Can you work these out from the model? Positions are in its coordinate system, mm. Face numbers are marked on the shaded views. Give positions to 0.01 mm unless a question says otherwise; leave off trailing zeros. Order: outer loops, then holes, each group sorted by start corner. A loop starts at its lowest first (then second) coordinate and runs counter-clockwise, first axis right, second up. Notation, with made-up numbers: M -31.5,-22.5 L -12.5,-22.5 A28 cw -12.5,-2.5 Z; hole C 47.5,-40 d6. An arc over 180 degrees is marked long. Write each question's results on one line, items separated by ' | '.
from build123d import *

# Parameters (mm, degrees)
SKETCH1_R               = 12
BOSS_EXTRUDE1_DEPTH     = 114.25
SKETCH2_R               = 11.565
CUT_EXTRUDE1_DEPTH      = 40
SKETCH3_R               = 3.3
CUT_EXTRUDE2_DEPTH      = 1
CUT_EXTRUDE2_DEPTH_BACK = 115.25


with BuildPart() as part:
    # Sketch1 → Boss-Extrude1 (new body)
    with BuildSketch(Plane(origin=(0, 0, 0), x_dir=(1, 0, 0), z_dir=(0, 1, 0))):
        Circle(SKETCH1_R)
    extrude(amount=BOSS_EXTRUDE1_DEPTH)

    # Sketch2 → Cut-Extrude1 (cut)
    with BuildSketch(Plane(origin=(0, 114.25, 0), x_dir=(1, 0, 0), z_dir=(0, 1, 0))):
        Circle(SKETCH2_R)
    extrude(amount=-CUT_EXTRUDE1_DEPTH, mode=Mode.SUBTRACT)

    # Sketch3 → Cut-Extrude2 (cut, two sides)
    with BuildSketch(Plane.XZ) as cut_extrude2_sk:
        Circle(SKETCH3_R)
    extrude(amount=CUT_EXTRUDE2_DEPTH, mode=Mode.SUBTRACT)
    extrude(cut_extrude2_sk.sketch, amount=-CUT_EXTRUDE2_DEPTH_BACK, mode=Mode.SUBTRACT)


solid = part.part
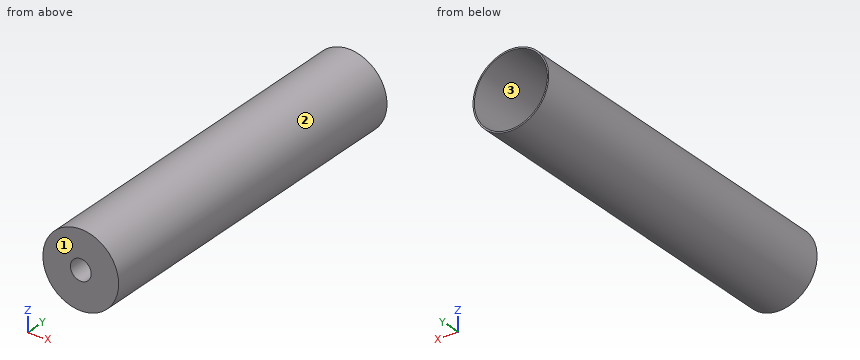
(1) I need wall thicknesses on L1, parallel to X at y = 100, z = 0 (3 decimals); L2, parallel to Y at x = -3.75, z = -6.75. Which ranges of each line are inside material? Lowest first, please. Write a range as from..to.
Data:
L1: x = -12..-11.565, 11.565..12 | L2: y = 0..74.25
(2) Imagine slicing it at C-C, the plane y = 79.5. Write out the boundary of the cut face in (x, z) (3 decimals), plus the area to 3 significant figures.
Data:
outline: C 0,0 d24; hole C 0,0 d23.13 | area: 32.2 mm2
(3) Imagine slicing it at A-A, the plane z = 0. Write out the boundary of the cut face in (x, y) (3 decimals).
Data:
outline: M -12,0 L -3.3,0 L -3.3,74.25 L -11.565,74.25 L -11.565,114.25 L -12,114.25 Z; M 3.3,0 L 12,0 L 12,114.25 L 11.565,114.25 L 11.565,74.25 L 3.3,74.25 Z
(4) Imagine slicing it at D-D, the plane z = 5. Write out the boundary of the cut face in (x, y), plus the area to 3 significant figures.
Data:
outline: M -10.91,0 L 10.91,0 L 10.91,114.25 L 10.43,114.25 L 10.43,74.25 L -10.43,74.25 L -10.43,114.25 L -10.91,114.25 Z | area: 1,660 mm2
(5) Will these pins go through, and if not, where does the flat tip stop? P1, Ø3, axis at x = -4.5, y = 37, coming from the +Z side; P2, Ø10, axis at y = 78, z = 9, coming from the -X side; P3, Ø1.5, axis at x = -9, y = 22, coming from the +Z side.
Data:
P1: stops at z = 11.62 | P2: stops at x = -11.31 | P3: stops at z = 8.71
(6) Imagine slicing it at B-B, the plane x = 0. Write out the boundary of the cut face in (y, z) (3 decimals), plus the area to 3 significant figures.
Data:
outline: M 0,-12 L 114.25,-12 L 114.25,-11.565 L 74.25,-11.565 L 74.25,-3.3 L 0,-3.3 Z; M 0,3.3 L 74.25,3.3 L 74.25,11.565 L 114.25,11.565 L 114.25,12 L 0,12 Z | area: 1,330 mm2
(7) We'd pull the mould along X, two halves only. Please class the marked faces 1, 2 and 3: +X half, -X half, draft (parallel to the pull), parting line (faces both ways), or undercut.
Data:
face 1: draft | face 2: parting line | face 3: undercut
